```python
from build123d import *

# Parameters (mm, degrees)
F0_W           = 5
F0_H           = 5.5
F0_W_2         = 5.5
F0_H_2         = 5
F0_W_3         = 51
F0_H_3         = 51
F1_DEPTH       = 190
F2_R           = 10
F3_R           = 25
F3_R_2         = 17.5
F3_R_3         = 20
F4_DEPTH       = 5
F5_D           = 5.1054
F5_DEPTH       = 12
F5_CSINK_D     = 10.4394
F5_CSINK_ANGLE = 82
F5_TIP         = 1.5338169022
F7_D           = 5.1054
F7_DEPTH       = 12
F7_CSINK_D     = 10.4394
F7_CSINK_ANGLE = 82
F7_TIP         = 1.5338169022
F6_R           = 20
F6_R_2         = 25
F6_R_3         = 17.5
F8_DEPTH       = 5
F10_DEPTH      = 2.5
F12_DEPTH      = 2.5


with BuildPart() as f1:
    # F0 (on Top) → F1 (new body)
    with BuildSketch(Plane.XY):
        Polygon((-33.5, 28), (-28, 28), (-28, 33.5), (-28, 36.5), (-36.5, 36.5), (-36.5, 28), align=None)
        Polygon((-28, 36.5), (-28, 33.5), (-23, 33.5), (-13, 33.5), (-13, 36.5), align=None)
        with Locations((-25.5, 30.75)):
            Rectangle(F0_W, F0_H)
        with Locations((-30.75, 25.5)):
            Rectangle(F0_W_2, F0_H_2)
        Polygon((-33.5, 23), (-33.5, 28), (-36.5, 28), (-36.5, 13), (-33.5, 13), align=None)
        Polygon((-23, 28), (-28, 28), (-28, 23), (-28, -30.5), (30.5, -30.5), (30.5, 28), align=None)
        Rectangle(F0_W_3, F0_H_3, mode=Mode.SUBTRACT)
    extrude(amount=F1_DEPTH)

    # F2
    f2_edges = [f1.edges().sort_by_distance(p)[0] for p in [
        (-36.5, 36.5, 95),
    ]]
    fillet(f2_edges, radius=F2_R)

    # F3 (on face) → F4 (cut, through all)
    with BuildSketch(Plane.XZ.offset(30.5)):
        with Locations((0, 100)):
            Circle(F3_R)
        with Locations((0, 165)):
            Circle(F3_R_2)
        with Locations((0, 30)):
            Circle(F3_R_3)
    extrude(amount=-F4_DEPTH, mode=Mode.SUBTRACT)

    # F5
    with Locations(Plane.XZ.offset(30.5)):
        with Locations((0, 140), (0, 60)):
            CounterSinkHole(F5_D / 2, F5_CSINK_D / 2, depth=F5_DEPTH, counter_sink_angle=F5_CSINK_ANGLE)
            with Locations((0, 0, -(F5_DEPTH + F5_TIP / 2))):  # 118° drill point
                Cone(0, F5_D / 2, F5_TIP, mode=Mode.SUBTRACT)

    # F7
    with Locations(Plane.YZ.offset(30.5)):
        with Locations((0, 130), (0, 50)):
            CounterSinkHole(F7_D / 2, F7_CSINK_D / 2, depth=F7_DEPTH, counter_sink_angle=F7_CSINK_ANGLE)
            with Locations((0, 0, -(F7_DEPTH + F7_TIP / 2))):  # 118° drill point
                Cone(0, F7_D / 2, F7_TIP, mode=Mode.SUBTRACT)

    # F6 (on face) → F8 (cut, through all)
    with BuildSketch(Plane.YZ.offset(30.5)):
        with Locations((0, 160)):
            Circle(F6_R)
        with Locations((0, 90)):
            Circle(F6_R_2)
        with Locations((0, 25)):
            Circle(F6_R_3)
    extrude(amount=-F8_DEPTH, mode=Mode.SUBTRACT)

    # F9 (on face) → F10 (cut, through all)
    with BuildSketch(Plane(origin=(-28, 0, 0), x_dir=(0, -1, 0), z_dir=(-1, 0, 0))):
        with BuildLine():
            Line((-23, 164.7979589711), (-23, 145.2020410289))
            ThreePointArc((-23, 145.2020410289), (5, 130.5051025722), (25, 155))
            ThreePointArc((25, 155), (5, 179.4948974278), (-23, 164.7979589711))
        make_face()
        with BuildLine():
            ThreePointArc((-23, 85.2020410289), (5, 70.5051025722), (25, 95))
            ThreePointArc((25, 95), (5, 119.4948974278), (-23, 104.7979589711))
            Line((-23, 104.7979589711), (-23, 85.2020410289))
        make_face()
        with BuildLine():
            ThreePointArc((25, 35), (5, 59.4948974278), (-23, 44.7979589711))
            Line((-23, 44.7979589711), (-23, 25.2020410289))
            ThreePointArc((-23, 25.2020410289), (5, 10.5051025722), (25, 35))
        make_face()
    extrude(amount=-F10_DEPTH, mode=Mode.SUBTRACT)

    # F11 (on face) → F12 (cut, through all)
    with BuildSketch(Plane(origin=(0, 28, 0), x_dir=(-1, 0, 0), z_dir=(0, 1, 0))):
        with BuildLine():
            ThreePointArc((23, 164.7979589711), (-25, 155), (23, 145.2020410289))
            Line((23, 145.2020410289), (23, 164.7979589711))
        make_face()
        with BuildLine():
            Line((23, 85.2020410289), (23, 104.7979589711))
            ThreePointArc((23, 104.7979589711), (-25, 95), (23, 85.2020410289))
        make_face()
        with BuildLine():
            Line((23, 25.2020410289), (23, 44.7979589711))
            ThreePointArc((23, 44.7979589711), (-25, 35), (23, 25.2020410289))
        make_face()
    extrude(amount=-F12_DEPTH, mode=Mode.SUBTRACT)


solid = f1.part
```
Geometry check sheet. Reference: the model listing, model coordinates, mm. A direction names the side the tool comes from. Coordinates: 2 decimals unless noted, no trailing zeros. One line per item, written item: value. Start each with the question number.
(1) Depth check by flat-ended pin: P1, Ø2.5, axis at y = 35.5, z = 115.5, coming from the +X side; P2, Ø6, axis at y = 0, z = 130, coming from the +X side; P3, Ø3, axis at x = 10, z = 128, coming from the +Y side. Enter the tip coordinate at first touch or a pass-through.
(2) Material ranges on line 1 (Z direction, x = 0, y = -27.4); line 2 (Z direction, x = 27.15, y = 0); line 3 (Y direction, x = -21.5, z = 131), recorded low to high. Write a range as [from, to].
(3) Tool access check on faces 4 (the flat face through (16, 28, 73)), 5 (the cylindrical face through (24.98, 26.77, 35.96)), 6 (the cylindrical face through (28.035, -5.42, 65.594)). Record the directions out of +Z, -Z, +X, -X, +Y, -Y that give a thin tool (end or side, any length) a straight path to the whole face; none if there is none.
(4) Cross-section at A-A on x = 15.5. Count the separate pieces of the cut face and the enclosed holes in it, plus the area to 3 significant figures.
(5) Mould release check, pull along Y, two halves, no side actions. Record for faces 1 (the cylindrical face through (28.04, -2.6, 179.83)), 2 (the flat face through (30.5, -8, 115)), 3 (the conical face through (1.98, -27.58, 141.81)): released by +Y, released by -Y, zero draft, split by the parting line, or undercut.
Results below:
1. P1: stops at x = -13
1. P2: stops at x = 27.95
1. P3: stops at y = 28
2. line 1: z = [0, 10], [50, 57.45], [62.55, 75], [125, 137.45], [142.55, 147.5], [182.5, 190]
2. line 2: z = [0, 7.5], [42.5, 47.45], [52.55, 65], [115, 127.45], [132.55, 140], [180, 190]
2. line 3: y = [-30.5, -25.5], [25.5, 28], [33.5, 36.5]
3. face 4: +Z, -Z, +X
3. face 5: none
3. face 6: +X
4. separate pieces: 8
4. enclosed holes: 0
4. area: 727 mm2
5. face 1: undercut
5. face 2: zero draft
5. face 3: released by -Y
